Build history of the part. All positions in model axes, mm. A direction names the side the tool comes from. Give positions to 0.01 mm unless a question says otherwise; leave off trailing zeros. Order: outer loops, then holes, each group sorted by start corner. A loop starts at its lowest first (then second) coordinate and runs counter-clockwise, first axis right, second up. Notation, with made-up numbers: (50.5, -37) - (85.5, -37) arc R14 cw to (85.5, -21) - close; hole circle Ø1 at (-15, 12.5). An arc over 180 degrees is marked (long way). One line per item, written item: value.
Autodesk Inventor part; units mm, degrees
ref_plane "YZ Plane" through (0, 0, 0) normal (1, 0, 0) x (0, 1, 0)
ref_plane "XZ Plane" through (0, 0, 0) normal (0, 1, 0) x (-1, 0, 0)
ref_plane "XY Plane" through (0, 0, 0) normal (0, 0, 1) x (1, 0, 0)
sketch "Szkic1" plane through (0, 0, 0) normal (0, 0, 1) x (1, 0, 0)
  line L0 (-0.9998, 0.9998) -> (-0.9998, 4.2541)
  ellipse E0 centre (0.0003, 1.0002) end of major axis (-0.707, 0.2928) minor radius 1 (-0.9998, 0.9998) -> (0, 0) ccw
  line L1 (0, 0) -> (40.8091, 0)
  ellipse E1 centre (40.809, 1.0002) end of major axis (41.1917, 0.0761) minor radius 1 (40.8091, 0) -> (41.5161, 0.2928) ccw
  line L2 (44.7924, 3.5691) -> (41.5161, 0.2928)
  ellipse E2 centre (44.0851, 4.2762) end of major axis (45.0091, 3.8935) minor radius 1 (44.7924, 3.5691) -> (45.0852, 4.2761) ccw
  line L3 (45.0852, 4.2761) -> (45.0852, 43.2644)
  ellipse E3 centre (44.5851, 43.2643) end of major axis (44.9388, 43.6179) minor radius 0.5 (45.0852, 43.2644) -> (44.5853, 43.7644) ccw
  line L4 (44.5853, 43.7644) -> (6.9989, 43.7644)
  ellipse E4 centre (7.0014, 35.7631) end of major axis (1.3428, 41.4217) minor radius 8 (6.9989, 43.7644) -> (-0.9998, 35.7656) ccw
  line L5 (-0.9998, 7.3746) -> (-0.9998, 35.7656)
  circle A0 centre (24.3209, 20.7644) radius 14
  circle A1 centre (8.8209, 36.2644) radius 3.4
  circle A2 centre (39.8209, 36.2644) radius 1.8356
  circle A3 centre (39.8209, 5.2644) radius 1.8356
  circle A4 centre (8.8209, 5.2644) radius 1.6
  line L6 (-0.9998, 7.3746) -> (-0.9998, 4.2541)
  circle A5 centre (25.4094, -15.2449) radius 1.5
  circle A6 centre (1.0095, -15.2313) radius 1.5
  arc A7 (28.4064, -20.7465) -> (29.4069, -19.7471) centre (28.4069, -19.7465) ccw
  line L7 (29.4106, -13.2471) -> (29.4069, -19.7471)
  line L8 (27.9114, -11.7463) -> (29.4106, -13.2471)
  line L9 (-1.4886, -11.7299) -> (27.9114, -11.7463)
  line L10 (-2.9894, -13.2291) -> (-1.4886, -11.7299)
  line L11 (-2.9931, -19.7291) -> (-2.9894, -13.2291)
  arc A8 (-2.9931, -19.7291) -> (-1.9936, -20.7296) centre (-1.9931, -19.7296) ccw
  line L12 (28.4064, -20.7465) -> (-1.9936, -20.7296)
  line L13 (-2.9894, -13.2291) -> (-0.9998, 0.9998)
  line L14 (29.4106, -13.2471) -> (41.5161, 0.2928)
  point P0 (0, 0)
  point P1 (0, 0)
  dimension "d15" = 0.5001
  dimension "d16" = 1.0002
  dimension "d17" = 1.0002
  dimension "d18" = 8.0024
  dimension "d19" = 1.0003
  dimension "d20" = 0.5
  dimension "d21" = 1
  dimension "d22" = 1
  dimension "d23" = 8
  dimension "d24" = 1
  dimension "d0" = 32.4
  dimension "d1" = 9
  dimension "d2" = 3.5
  dimension "d3" = 3.5
  dimension "d4" = 4
  dimension "d5" = 4
  dimension "d6" = 1
  dimension "d7" = 3
  dimension "d8" = 135
  dimension "d9" = 4.5962
  dimension "d10" = 27.5065
  dimension "d11" = 3.6713
  dimension "d12" = 28
  dimension "d13" = 6.8
  dimension "d14" = 3.2
  dimension "d25" = 135
  dimension "d26" = 46.0851
  dimension "d27" = 43.7644
  dimension "d28" = 45.0852
  dimension "d29" = 29.1492
  dimension "d30" = 43.7644
  dimension "d31" = 4.2761
  dimension "d32" = 3.5691
  dimension "d33" = 5.2644
  dimension "d34" = 26.6344
  dimension "d35" = 5.2644
  dimension "d36" = 4.7141
  dimension "d37" = 20.7644
  dimension "d38" = 26.6344
  dimension "d39" = 20.7644
  dimension "d40" = 26.6344
  dimension "d41" = 36.2644
  dimension "d42" = 48.5547
  dimension "d43" = 36.2644
  dimension "d44" = 26.6344
  dimension "d45" = 45.0852
  dimension "d46" = 29.1492
  dimension "d47" = 35.0709
  dimension "d48" = 32.8644
  dimension "d55" = 11.8
  dimension "d56" = 17
extrude "Wyciągnięcie proste1" add sketch "Szkic1" along normal blind 2.5
fillet "Zaokrąglenie1" radius 10 3 edges at (-2.9931, -19.7291, 1.25) (-0.9998, 0.9998, 1.25) (29.4106, -13.2471, 1.25)
properties part number "3DP_ABS_E3D_Titan_Mounting_Plate"
(1) Pin check, flat tip, straight feed: P1, Ø3.5, axis at x = 25.41, y = -15.24, coming from the +Z side. Stop position of the tip, or through.
Completed:
P1: z = 2.5
(2) Pull direction Y, two halves, no side cores. Call faces 3 (the face through (21, 5, 0)), 4 (the face through (31.85, 8.96, 1.23)), 5 (the face through (43.177, 1.954, 1.232)): +Y half, -Y half, draft (parallel to the pull), parting line (faces both ways), or undercut.
Completed:
face 3: draft
face 4: undercut
face 5: -Y half
(3) Slice it at A-A, the plane x = 21.5. Give the cut face in (y, z), and give its area (3 significant figures).
Completed:
outline: (-20.74, 0) - (7.05, 0) - (7.05, 2.5) - (-20.74, 2.5) - close; (34.48, 0) - (43.76, 0) - (43.76, 2.5) - (34.48, 2.5) - close
area: 92.7 mm²
(4) Slice it at B-B, the plane y = 8.5. Give the cut face in (x, z), and give its area (3 significant figures).
Completed:
outline: (-1, 0) - (17.57, 0) - (17.57, 2.5) - (-1, 2.5) - close; (31.07, 0) - (45.09, 0) - (45.09, 2.5) - (31.07, 2.5) - close
area: 81.5 mm²
(5) Slice it at C-C, the plane z = 1.85. Count the separate pieces of the cut face and the enclosed holes in it, and give its area (3 significant figures).
Completed:
separate pieces: 1
enclosed holes: 7
area: 2,040 mm²
(6) 3-axis set-ups, long thin cutter, end or side, ignore diameter. For faces 1 (the face through (-1, 18, 1)), 2 (the face through (40.67, 37.89, 1.23)): which of +Z, -Z, +X, -X, +Y, -Y reach the whole face in a straight line?
Completed:
face 1: +Z, -Z, -X, +Y
face 2: +Z, -Z
(7) Drill centre lines: line 1 (Y direction, x = 9, z = 2.2); line 2 (X direction, y = -14, z = 0.75); line 3 (X direction, y = -17, z = 0.5). Where is each one in solid material? Low to high.
Completed:
line 1: -20.74 to 3.67, 6.85 to 32.87, 39.66 to 43.76
line 2: -2.99 to 0.15, 1.87 to 24.57, 26.25 to 29.89
line 3: -2.99 to 29.41
